Input: part model. Units: mm. Frame: model coordinates. A direction names the side the tool comes from. Coordinates: 2 decimals unless noted, no trailing zeros. Use one line per item in the form item = value.
Autodesk Inventor part; units mm, degrees
ref_plane "YZ Plane" through (0, 0, 0) normal (1, 0, 0) x (0, 1, 0)
ref_plane "XZ Plane" through (0, 0, 0) normal (0, 1, 0) x (-1, 0, 0)
ref_plane "XY Plane" through (0, 0, 0) normal (0, 0, 1) x (1, 0, 0)
sketch "Sketch1" plane through (0, 0, 0) normal (0, 1, 0) x (-1, 0, 0)
  line L0 (0, 25.4) -> (25.4, 25.4)
  line L1 (25.4, 25.4) -> (25.4, 0)
  line L2 (25.4, 0) -> (0, 0)
  line L3 (0, 0) -> (0, 25.4)
  line L4 (22.225, 22.225) -> (3.175, 22.225)
  line L5 (3.175, 22.225) -> (3.175, 3.175)
  line L6 (3.175, 3.175) -> (22.225, 3.175)
  line L7 (22.225, 3.175) -> (22.225, 22.225)
  dimension "d0" = 25.4
  dimension "d1" = 25.4
  dimension "d2" = 3.175
extrude "Extrusion1" add sketch "Sketch1" along normal blind 660.4
sketch "Sketch2" plane through (-25.4, 0, 25.4) normal (0, 0, 1) x (1, 0, 0)
  circle A0 centre (12.7, 534.8581) radius 3.302
  circle A1 centre (12.7, 491.7722) radius 3.302
  circle A2 centre (12.7, 448.6863) radius 3.302
  circle A3 centre (12.7, 405.6004) radius 3.302
  circle A4 centre (12.7, 362.5144) radius 3.302
  circle A5 centre (12.7, 319.4285) radius 3.302
  circle A6 centre (12.7, 276.3426) radius 3.302
  circle A7 centre (12.7, 233.2567) radius 3.302
  circle A8 centre (12.7, 190.1707) radius 3.302
  circle A9 centre (12.7, 147.0848) radius 3.302
  circle A10 centre (12.7, 103.9989) radius 3.302
  circle A11 centre (12.7, 125.5419) radius 3.302
  circle A12 centre (12.7, 168.6278) radius 3.302
  circle A13 centre (12.7, 211.7137) radius 3.302
  circle A14 centre (12.7, 254.7996) radius 3.302
  circle A15 centre (12.7, 297.8856) radius 3.302
  circle A16 centre (12.7, 340.9715) radius 3.302
  circle A17 centre (12.7, 384.0574) radius 3.302
  circle A18 centre (12.7, 427.1433) radius 3.302
  circle A19 centre (12.7, 470.2293) radius 3.302
  circle A20 centre (12.7, 513.3152) radius 3.302
  circle A21 centre (12.7, 556.4011) radius 3.302
  line L0 (25.4, 25.4) -> (0, 25.4)
  line L1 (25.4, 25.4) -> (25.4, 635)
  line L2 (0, 635) -> (25.4, 635)
  line L3 (0, 25.4) -> (0, 635)
extrude "Extrusion2" cut sketch "Sketch2" against normal through all contours A1 | A3 | A7 | A10 | A12 | A14 | A18 | A21
sketch "Sketch3" plane through (-25.4, 0, 0) normal (-1, 0, 0) x (0, 0, 1)
  line L0 (25.4, 0) -> (25.4, 660.4)
  line L1 (0, 0) -> (0, 660.4)
  line L2 (0, 556.4011) -> (25.4, 556.4011) construction
  line L3 (0, 405.6004) -> (25.4, 405.6004) construction
  line L4 (0, 254.7996) -> (25.4, 254.7996) construction
  line L5 (0, 103.9989) -> (25.4, 103.9989) construction
  line L6 (12.7, 569.1011) -> (12.7, 524.6511) construction
  line L7 (12.7, 435.7629) -> (12.7, 375.4379) construction
  line L8 (12.7, 277.0246) -> (12.7, 232.5746) construction
  line L9 (12.7, 135.7489) -> (12.7, 91.2989) construction
  circle A0 centre (12.7, 569.1011) radius 3.302
  circle A1 centre (12.7, 524.6511) radius 3.302
  circle A2 centre (12.7, 435.7629) radius 3.302
  circle A3 centre (12.7, 375.4379) radius 3.302
  circle A4 centre (12.7, 277.0246) radius 3.302
  circle A5 centre (12.7, 232.5746) radius 3.302
  circle A6 centre (12.7, 135.7489) radius 3.302
  circle A7 centre (12.7, 91.2989) radius 3.302
  line L10 (0, 330.2) -> (25.4, 330.2) construction
  line L11 (12.7, 360.3625) -> (12.7, 300.0375) construction
  circle A8 centre (12.7, 360.3625) radius 3.302
  circle A9 centre (12.7, 300.0375) radius 3.302
  line L12 (0, 660.4) -> (25.4, 660.4)
  line L13 (0, 113.5239) -> (25.4, 113.5239) construction
  line L14 (25.4, 0) -> (0, 0)
  line L15 (0, 546.8761) -> (25.4, 546.8761) construction
  circle A10 centre (12.7, 12.7) radius 3.302
  circle A11 centre (12.7, 34.925) radius 3.302
  circle A12 centre (12.7, 50.8) radius 3.302
  line L16 (22.225, 553.0991) -> (22.225, 559.7031)
  line L17 (22.225, 402.2984) -> (22.225, 408.9024)
  line L18 (22.225, 251.4976) -> (22.225, 258.1016)
  line L19 (22.225, 100.6969) -> (22.225, 107.3009)
  circle A13 centre (12.7, 647.7) radius 3.302
  circle A14 centre (12.7, 625.475) radius 3.302
  circle A15 centre (12.7, 609.6) radius 3.302
  point P0 (12.7, 254.7996)
  point P1 (12.7, 405.6004)
  point P2 (12.7, 330.2)
  point P3 (12.7, 113.5239)
  point P4 (12.7, 546.8761)
  point P5 (22.225, 556.4011)
  point P6 (22.225, 405.6004)
  point P7 (22.225, 254.7996)
  point P8 (22.225, 103.9989)
  dimension "d7" = 44.45
  dimension "d8" = 60.325
  dimension "d9" = 44.45
  dimension "d10" = 44.45
  dimension "d11" = 6.604
  dimension "d12" = 6.604
  dimension "d13" = 6.604
  dimension "d14" = 6.604
  dimension "d15" = 6.604
  dimension "d16" = 6.604
  dimension "d17" = 6.604
  dimension "d18" = 6.604
  dimension "d21" = 60.325
  dimension "d22" = 6.604
  dimension "d23" = 6.604
  dimension "d27" = 9.525
  dimension "d28" = 9.525
extrude "Extrusion3" cut sketch "Sketch3" against normal blind 25.4 contours A0 | A1 | A6 | A7 | A8 | A9 | A10 | A11 | A12 | A13 | A14 | A15
sketch "Sketch4" plane through (0, 0, 25.4) normal (1, 0, 0) x (0, 0, -1)
  line L0 (25.4, 0) -> (25.4, 660.4)
  line L1 (0, 0) -> (0, 660.4)
  line L2 (0, 330.2) -> (25.4, 330.2) construction
  line L3 (12.7, 374.65) -> (12.7, 285.75) construction
  circle A0 centre (12.7, 374.65) radius 3.302 construction
  circle A1 centre (12.7, 285.75) radius 3.302 construction
  circle A2 centre (12.7, 393.7) radius 3.302
  circle A3 centre (12.7, 412.75) radius 3.302
  circle A4 centre (12.7, 431.8) radius 3.302
  circle A5 centre (12.7, 450.85) radius 3.302
  circle A6 centre (12.7, 469.9) radius 3.302
  circle A7 centre (12.7, 266.7) radius 3.302
  circle A8 centre (12.7, 247.65) radius 3.302
  circle A9 centre (12.7, 228.6) radius 3.302
  circle A10 centre (12.7, 209.55) radius 3.302
  circle A11 centre (12.7, 190.5) radius 3.302
  circle A12 centre (12.7, 488.95) radius 3.302
  circle A13 centre (12.7, 171.45) radius 3.302
  circle A14 centre (12.7, 360.3625) radius 3.302 construction
  circle A15 centre (12.7, 300.0375) radius 3.302 construction
  circle A16 centre (12.7, 319.0875) radius 3.302
  circle A17 centre (12.7, 341.3125) radius 3.302
  line L4 (12.7, 379.4125) -> (12.7, 374.65) construction
  line L5 (12.7, 285.75) -> (12.7, 280.9875) construction
  circle A18 centre (12.7, 379.4125) radius 3.302
  circle A19 centre (12.7, 280.9875) radius 3.302
  point P0 (12.7, 330.2)
  dimension "d33" = 88.9
  dimension "d34" = 6.604
  dimension "d37" = 19.05
  dimension "d44" = 19.05
  dimension "d51" = 19.05
  dimension "d52" = 19.05
  dimension "d53" = 19.05
  dimension "d54" = 19.05
extrude "Extrusion4" cut sketch "Sketch4" against normal blind 25.4
equation "\"d9\" = d7"
equation "\"d10\" = d7"
equation "\"d12\" = d11"
equation "\"d13\" = d11"
equation "\"d14\" = d11"
equation "\"d15\" = d11"
equation "\"d16\" = d11"
equation "\"d17\" = d11"
equation "\"d18\" = d11"
equation "\"d21\" = d8"
equation "\"d22\" = d11"
equation "\"d23\" = d11"
equation "\"d27\" = d28"
equation "\"d52\" = d51"
equation "\"d53\" = d51"
equation "\"d54\" = d51"
properties part number "Chassis Part1 (26x28)" material "Aluminum 6061"
(1) Pull-direction query (X, two-part tool) for faces 1 (the flat face through (-13, 326, 3.175)), 2 (the flat face through (0, 326, 13)), 3 (the flat face through (-3.175, 326, 13)), 4 (the flat face through (-13, 326, 25.4)); classes: pulls with the +X half, pulls with the -X half, needs draft (parallel to the pull), parting line crosses it, or undercut.
Computed:
face_1 = undercut
face_2 = pulls with the +X half
face_3 = undercut
face_4 = needs draft
(2) Set-up query: faces 5 (the flat face through (-22.225, 326, 13)), 6 (the flat face through (-24, 0, 13)). Return all of +Z, -Z, +X, -X, +Y, -Y with unobstructed straight access to the full face (end or side cutting, diameter ignored); none if empty.
Computed:
face_5 = +Y, -Y
face_6 = +Z, -Z, +X, -X, -Y
(3) Line query: probe 1 along Z at (x, y) = (-4.75, 146) (3 decimals); probe 2 along X at (y, z) = (476, 4.25) (3 decimals); probe 3 along Z at (x, y) = (-23.8, 431.8). Output: solid intervals per line, ascending.
Computed:
probe_1 = 0 to 3.175, 22.225 to 25.4
probe_2 = -25.4 to -22.225, -3.175 to 0
probe_3 = 0 to 9.4, 16 to 25.4
(4) First-contact query: pin 1 Ø1 at (y, z) = (580, 16.5) entering from +X; pin 2 Ø4 at (y, z) = (190.5, 12.7) entering from +X. Flat tips, straight axial feed; report the tip coordinate or a pass-through.
Computed:
pin_1 = 0
pin_2 = through
